Check sheet for the modelled part. Datum: model origin and axes. Units: mm. A direction names the side the tool comes from. Give positions to 0.01 mm unless a question says otherwise; leave off trailing zeros. Loops run counter-clockwise (first coordinate to the right, second up) from the corner with the lowest first, then second, coordinate; pieces in that order, holes last.
```python
from build123d import *

# Parameters (mm, degrees)
SKETCH1_R               = 3.5
SKETCH1_R_2             = 2
BOSS_EXTRUDE1_DEPTH     = 10
SKETCH2_W               = 7
SKETCH2_H               = 7
BOSS_EXTRUDE2_DEPTH     = 8
SKETCH3_W               = 4
SKETCH3_H               = 10
CUT_EXTRUDE1_DEPTH      = 4.5
CUT_EXTRUDE1_DEPTH_BACK = 4.5
SKETCH4_R               = 2
CUT_EXTRUDE2_DEPTH      = 4.5
CUT_EXTRUDE2_DEPTH_BACK = 4.5


with BuildPart() as part:
    # Sketch1 → Boss-Extrude1 (new body)
    with BuildSketch(Plane.XY):
        Circle(SKETCH1_R)
        Circle(SKETCH1_R_2, mode=Mode.SUBTRACT)
    extrude(amount=BOSS_EXTRUDE1_DEPTH)

    # Sketch2 → Boss-Extrude2 (add)
    with BuildSketch(Plane.XY):
        Rectangle(SKETCH2_W, SKETCH2_H)
    extrude(amount=-BOSS_EXTRUDE2_DEPTH)

    # Sketch3 → Cut-Extrude1 (cut, two sides)
    with BuildSketch(Plane(origin=(0, 0, 0), x_dir=(1, 0, 0), z_dir=(0, 1, 0))) as cut_extrude1_sk:
        with Locations((0, 6)):
            Rectangle(SKETCH3_W, SKETCH3_H)
    extrude(amount=CUT_EXTRUDE1_DEPTH, mode=Mode.SUBTRACT)
    extrude(cut_extrude1_sk.sketch, amount=-CUT_EXTRUDE1_DEPTH_BACK, mode=Mode.SUBTRACT)

    # Sketch4 → Cut-Extrude2 (cut, two sides)
    with BuildSketch(Plane(origin=(0, 0, 0), x_dir=(0, 0, -1), z_dir=(1, 0, 0))) as cut_extrude2_sk:
        with Locations((4.5, 0)):
            Circle(SKETCH4_R)
    extrude(amount=CUT_EXTRUDE2_DEPTH, mode=Mode.SUBTRACT)
    extrude(cut_extrude2_sk.sketch, amount=-CUT_EXTRUDE2_DEPTH_BACK, mode=Mode.SUBTRACT)


solid = part.part
```
(1) Section check C-C on y = 0.75. Record the boundary of the cut face in (x, z), plus the area to 3 significant figures.
(2) Section check A-A on z = -2. Record the boundary of the cut face in (x, y), plus the area to 3 significant figures.
(3) Section check B-B on z = -4.5. Record the boundary of the cut face in (x, y), plus the area to 3 significant figures.
(4) Section check D-D on x = 1. Record the boundary of the cut face in (y, z).
(5) Gauge pin test, flat ends, axial feed: pin 1 Ø1.1 at (x, y) = (-1, -1) entering from +Z; pin 2 Ø1.5 at (x, y) = (-1, 2) entering from -Z. Record the tip position at first contact, or that the pin passes through.
(6) Access from +Z, -Z, +X, -X, +Y, -Y to the whole of each face (thin tool, end or side, straight path). Record for faces 4 (the face through (2, -2, -3)), 5 (the face through (-3, -3, 0)), 6 (the face through (3.233, -1.341, 4.93)), 7 (the face through (3, 3, 0)).
(7) Release check for a two-part mould opening along Y. For faces 1 (the face through (2.74, 0.088, -2.502)), 2 (the face through (-2.4, -3.5, -3.9)), 3 (the face through (3, -3, 0)) record: pulls with the +Y half, pulls with the -Y half, needs draft (parallel to the pull), parting line crosses it, or undercut.
(8) Material ranges on line 1 (Y direction, x = 0, z = 2.5); line 2 (Z direction, x = 2.75, y = 0), recorded low to high.
Computed values:
1. outline: (-3.5, -8) - (-2, -8) - (-2, -6.35) - (-3.5, -6.35) - close; (-3.5, -2.65) - (-2, -2.65) - (-2, -1) - (2, -1) - (2, -2.65) - (3.5, -2.65) - (3.5, 0) - (3.42, 0) - (3.42, 10) - (1.85, 10) - (1.85, 0) - (-1.85, 0) - (-1.85, 10) - (-3.42, 10) - (-3.42, 0) - (-3.5, 0) - close; (2, -8) - (3.5, -8) - (3.5, -6.35) - (2, -6.35) - close
1. area: 48.2 mm2
2. outline: (-3.5, -3.5) - (-2, -3.5) - (-2, 3.5) - (-3.5, 3.5) - close; (2, -3.5) - (3.5, -3.5) - (3.5, 3.5) - (2, 3.5) - close
2. area: 21.0 mm2
3. outline: (-3.5, -3.5) - (-2, -3.5) - (-2, -2) - (-3.5, -2) - close; (-3.5, 2) - (-2, 2) - (-2, 3.5) - (-3.5, 3.5) - close; (2, -3.5) - (3.5, -3.5) - (3.5, -2) - (2, -2) - close; (2, 2) - (3.5, 2) - (3.5, 3.5) - (2, 3.5) - close
3. area: 9.00 mm2
4. outline: (-3.5, -1) - (3.5, -1) - (3.5, 0) - (3.35, 0) - (3.35, 10) - (1.73, 10) - (1.73, 0) - (-1.73, 0) - (-1.73, 10) - (-3.35, 10) - (-3.35, 0) - (-3.5, 0) - close
5. pin 1: stops at z = 0
5. pin 2: stops at z = -1
6. face 4: -Z, +Y, -Y
6. face 5: +Z, -X, -Y
6. face 6: +Z
6. face 7: +Z, +X, +Y
7. face 1: undercut
7. face 2: pulls with the -Y half
7. face 3: needs draft
8. line 1: y = -3.5 to -2, 2 to 3.5
8. line 2: z = -8 to -6.5, -2.5 to 10
